Here's how the part is built. I have some questions about the finished solid (model axes, mm). A direction names the side the tool comes from. Round coordinates to 2 decimals unless told otherwise and drop trailing zeros. Order: outer loops, then holes, each group sorted by start corner. A loop starts at its lowest first (then second) coordinate and runs counter-clockwise, first axis right, second up. Notation, with made-up numbers: (29.5, -20.75) -> (70.5, -20.75) arc R31 ccw to (70.5, 11.25) -> close; hole circle Ø3 at (-16, 10.25). An arc over 180 degrees is marked (long way). Use a Markdown table: item, result. Add a question column.
(1) I want a section at D-D, the plane y = -86. Please give me the cut outline in (x, z), then the cut area to 3 significant figures.
(2) I want a section at B-B, the plane y = 132. Please give me the cut outline in (x, z).
(3) I'm going to push flat-ended pins straight in: P1, Ø6.5, axis at x = 147.6, y = 56.35, coming from the +Z side; P2, Ø3, axis at y = 33.5, z = 1.5, coming from the -X side; P3, Ø2.5, axis at y = -188.5, z = 2, coming from the -X side; P4, Ø2.5, axis at y = -182, z = 3.5, coming from the +X side. Where does each tip first touch, or does it pass through?
(4) If I drill on probe 1 along Y at (x, z) = (10, 3.9); probe 2 along Y at (x, z) = (13, 1.5); probe 3 along X at (y, z) = (53.5, 3), over which ranges is the centre line in solid material (lowest first)?
(5) On a 3-axis mill with a long thin cutter (end or side, diameter ignored), from which of +Z, -Z, +X, -X, +Y, -Y can I reach the whole of each face in a straight line? I mean faces 1 (the face through (-25.23, -14.3, 2.54)), 2 (the face through (-152.65, 151.6, 2.54)), 3 (the face through (-181.56, 52.86, 2.54)), 4 (the face through (136.558, 130.803, 2.535)), 5 (the face through (-139.599, -78.208, 2.465)). Say none if no direction works.
(6) I want a section at C-C, the plane z = 2.15. Give the number of separate pieces and of enclosed holes in the cut face, then the cut area to 3 significant figures.
(7) Thinking about a two-plate mould opening in Y: for faces 6 (the face through (153, 151, 3)), 7 (the face through (138.88, 79.45, 2.54)), 8 (the face through (-137.14, 131.14, 2.54)), 9 (the face through (-50, 19, 5)), which applies, pulls with the +Y half, pulls with the -Y half, needs draft (parallel to the pull), parting line crosses it, or undercut?
(8) I want a section at A-A, the plane x = -137. Please give me the cut outline in (y, z).
from build123d import *

# Parameters (mm, degrees)
EXTRUDE_1_DEPTH          = 5
CUT_EXTRUDE_1_DEPTH      = 424.349737215
M5X0_8_1_D               = 4.2
HOLE_WIZARD_M4_1_D       = 4.3
PATTERN_CIRCULAR_1_COUNT = 3
CUT_EXTRUDE_2_DEPTH      = 298.372381591


with BuildPart() as part:
    # Sketch 1 → Extrude 1 (new body)
    with BuildSketch(Plane.XY):
        Polygon((0, -320), (277.128129211, 160), (-277.128129211, 160), align=None)
    extrude(amount=EXTRUDE_1_DEPTH)

    # Sketch 6 → Cut-Extrude 1 (cut, through all)
    with BuildSketch(Plane.XY.offset(5)):
        Polygon((-64.663230149, -208), (-45, -208), (-45, -160), (45, -160), (45, -208), (64.663230149, -208), (0, -320), align=None)
    cut_extrude_1 = extrude(amount=-CUT_EXTRUDE_1_DEPTH, mode=Mode.SUBTRACT)

    # M5x0.8 _1 (through all)
    with Locations(Plane.XY.offset(5)):
        with Locations((25, -156), (-25, -156)):
            m5x0_8_1 = Hole(M5X0_8_1_D / 2)

    # Hole Wizard M4 _1 (through all)
    with Locations(Plane.XY.offset(5)):
        with Locations((10, -93), (-10, -93)):
            hole_wizard_m4_1 = Hole(HOLE_WIZARD_M4_1_D / 2)

    # Pattern Circular 1: Cut-Extrude 1, M5x0.8 _1, Hole Wizard M4 _1 ×3 about axis
    pattern_circular_1_axis = Axis((0, 0, 0), (0, 0, 1))
    add([cut_extrude_1.rotate(pattern_circular_1_axis, i * 360 / PATTERN_CIRCULAR_1_COUNT) for i in range(1, PATTERN_CIRCULAR_1_COUNT)], mode=Mode.SUBTRACT)
    add([m5x0_8_1.rotate(pattern_circular_1_axis, i * 360 / PATTERN_CIRCULAR_1_COUNT) for i in range(1, PATTERN_CIRCULAR_1_COUNT)], mode=Mode.SUBTRACT)
    add([hole_wizard_m4_1.rotate(pattern_circular_1_axis, i * 360 / PATTERN_CIRCULAR_1_COUNT) for i in range(1, PATTERN_CIRCULAR_1_COUNT)], mode=Mode.SUBTRACT)

    # Sketch 11 → Cut-Extrude 2 (cut, through all)
    with BuildSketch(Plane.XY.offset(5)):
        Polygon((33.486315613, 0), (16.743157806, 29), (-16.743157806, 29), (-33.486315613, 0), (-16.743157806, -29), (16.743157806, -29), align=None)
    extrude(amount=-CUT_EXTRUDE_2_DEPTH, mode=Mode.SUBTRACT)


solid = part.part
Taken from the geometry:
| question | item | result |
|---|---|---|
| 1 | outline | (-135.1, 0) -> (135.1, 0) -> (135.1, 5) -> (-135.1, 5) -> close |
| 1 | area | 1,350 mm2 |
| 2 | outline | (-138.63, 0) -> (138.63, 0) -> (138.63, 5) -> (-138.63, 5) -> close |
| 3 | P1 | stops at z = 5 |
| 3 | P2 | stops at x = -204.96 |
| 3 | P3 | stops at x = -76.64 |
| 3 | P4 | stops at x = 80.4 |
| 4 | probe 1 | y = -160 to -95.15, -90.85 to -29, 29 to 160 |
| 4 | probe 2 | y = -160 to -29, 29 to 160 |
| 4 | probe 3 | x = -209.29 to -182.66, -153.86 to -76.91, -74.17 to 74.17, 76.91 to 153.86, 182.66 to 209.29 |
| 5 | face 1 | +Z, -Z |
| 5 | face 2 | +Z, -Z, -X, +Y |
| 5 | face 3 | +Z, -Z, +Y |
| 5 | face 4 | +Z, -Z, +X |
| 5 | face 5 | +Z, -Z, -X, -Y |
| 6 | separate pieces | 1 |
| 6 | enclosed holes | 13 |
| 6 | area | 95,300 mm2 |
| 7 | face 6 | pulls with the +Y half |
| 7 | face 7 | undercut |
| 7 | face 8 | undercut |
| 7 | face 9 | needs draft |
| 8 | outline | (-82.71, 0) -> (82.71, 0) -> (82.71, 5) -> (-82.71, 5) -> close; (131.06, 0) -> (160, 0) -> (160, 5) -> (131.06, 5) -> close |
